Design review of the part built by this model. Coordinates are the model's own, in mm. Face numbers are marked on the shaded views. A direction names the side the tool comes from. Round coordinates to 2 decimals unless told otherwise and drop trailing zeros. Loops run counter-clockwise (first coordinate to the right, second up) from the corner with the lowest first, then second, coordinate; pieces in that order, holes last. Notation, with made-up numbers: M 85,69.5 L 102,69.5 A24 ccw 102,99.5 Z; hole C -21,28.5 d6. An arc over 180 degrees is marked long. Use a Markdown table: item, result.
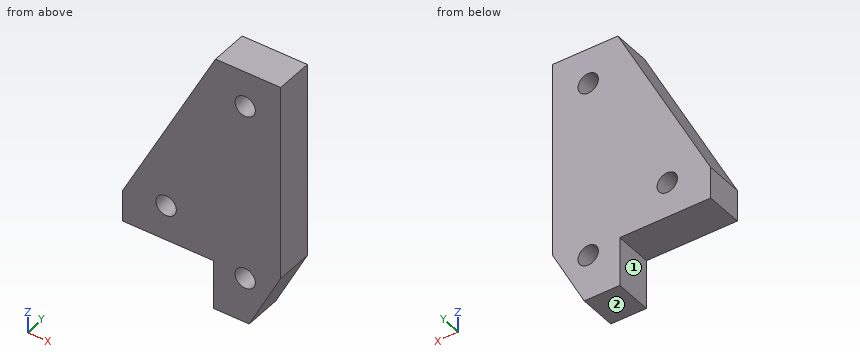
from build123d import *

# Parameters (mm, degrees)
F1_DEPTH = 19
F2_D     = 10.3
F4_D     = 10.3


with BuildPart() as f1:
    # F0 (on Front) → F1 (new body)
    with BuildSketch(Plane.XZ):
        Polygon((80, 168), (47, 168), (0, 78), (0, 62), (46, 62), (46, 37), (64.0441176471, 37), (80, 68), align=None)
    extrude(amount=F1_DEPTH)

    # F2 (through all)
    with Locations(Plane(origin=(0, 0, 0), x_dir=(1, 0, 0), z_dir=(0, 1, 0))):
        with Locations((62, -150)):
            Hole(F2_D / 2)

    # F4 (through all)
    with Locations(Plane.XZ.offset(19)):
        with Locations((22, 80), (62, 60)):
            Hole(F4_D / 2)


solid = f1.part
1. Take a section at D-D on x = 23.5. Give the boundary of the cut face in (y, z).
Check values:
| item | result |
|---|---|
| outline | M -19,62 L 0,62 L 0,75.07 L -19,75.07 Z; M -19,84.93 L 0,84.93 L 0,123 L -19,123 Z |
2. Take a section at A-A on z = 150. Give the boundary of the cut face in (x, y).
Check values:
| item | result |
|---|---|
| outline | M 37.6,-19 L 56.85,-19 L 56.85,0 L 37.6,0 Z; M 67.15,-19 L 80,-19 L 80,0 L 67.15,0 Z |
3. Wall thickness on line 1 along Z through (x, y) = (62, -14); line 2 along Z through (x, y) = (64, -0.75); line 3 along Z through (x, y) = (22, -11): over which ranges is each line inside the solid? List them lowest first. Write a range as from..to.
Check values:
| item | result |
|---|---|
| line 1 | z = 37..54.85, 65.15..144.85, 155.15..168 |
| line 2 | z = 37..55.25, 64.75..145.25, 154.75..168 |
| line 3 | z = 62..74.85, 85.15..120.13 |
4. Take a section at C-C on y = -4.75. Give the boundary of the cut face in (x, z), and give its area (3 significant figures).
Check values:
| item | result |
|---|---|
| outline | M 0,62 L 46,62 L 46,37 L 64.04,37 L 80,68 L 80,168 L 47,168 L 0,78 Z; hole C 22,80 d10.3; hole C 62,60 d10.3; hole C 62,150 d10.3 |
| area | 6,720 mm² |
5. Insertion check: pin 1 (8 mm diameter, centred on x = 62, z = 60, fed in from -Y); pin 2 (6 mm diameter, centred on y = -2.5, z = 95.5, fed in from -X); pin 3 (5.5 mm diameter, centred on y = -9, z = 53, fed in from -X); pin 4 (1.5 mm diameter, centred on x = 10, y = -12, fed in from -Z). Each pin has a flat end and moves straight along its axis. Give the tip position at first contact, or say it passes through.
Check values:
| item | result |
|---|---|
| pin 1 | passes through |
| pin 2 | stops at x = 7.57 |
| pin 3 | stops at x = 46 |
| pin 4 | stops at z = 62 |
6. Take a section at B-B on x = 62. Give the boundary of the cut face in (y, z), and give its area (3 significant figures).
Check values:
| item | result |
|---|---|
| outline | M -19,37 L 0,37 L 0,54.85 L -19,54.85 Z; M -19,65.15 L 0,65.15 L 0,144.85 L -19,144.85 Z; M -19,155.15 L 0,155.15 L 0,168 L -19,168 Z |
| area | 2,100 mm² |
7. Machinability: for the marked faces 1 and 2, which of the approach directions +Z, -Z, +X, -X, +Y, -Y give a long, thin tool a straight path to every point of the face, cutting with its end or side? Answer none if there is none.
Check values:
| item | result |
|---|---|
| face 1 | -Z, -X, +Y, -Y |
| face 2 | -Z, +X, -X, +Y, -Y |
